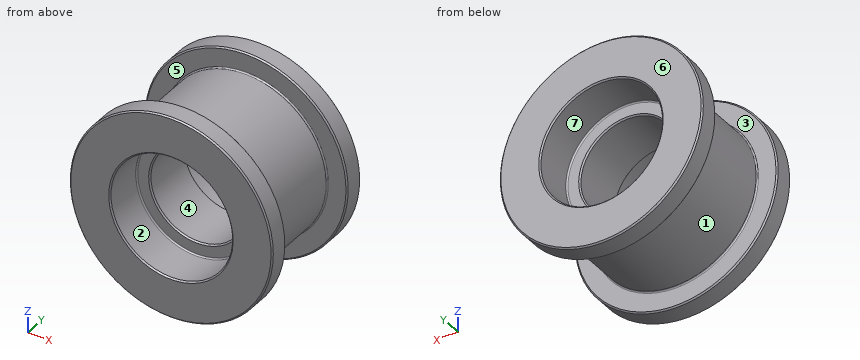
from build123d import *

# Parameters (mm, degrees)
ZKOSEN_1_SIZE = 0.1
ZAOBLIT1_R    = 0.1


with BuildPart() as part:
    # Skica1 → Rotovat1 (revolve)
    with BuildSketch(Plane.XY, mode=Mode.PRIVATE) as rotovat1_sk:
        Polygon((4.5, 10), (7.5, 10), (7.5, 8.5), (6, 8.5), (6, 1.5), (7.5, 1.5), (7.5, 0), (4.5, 0), (4.5, 3), (3.5, 3), (3.5, 7), (4.5, 7), align=None)
    revolve(rotovat1_sk.sketch.rotate(Axis((0, 0, 0), (0, -1, 0)), 90), axis=Axis((0, 0, 0), (0, -1, 0)))

    # Zkosení1
    zkosen_1_edges = [part.edges().sort_by_distance(p)[0] for p in [
        (0, 3, -3.5),
        (0, 0, -4.5),
        (0, 0, -7.5),
        (0, 1.5, -7.5),
        (0, 8.5, -7.5),
        (0, 10, -7.5),
        (0, 10, -4.5),
        (0, 7, -3.5),
    ]]
    chamfer(zkosen_1_edges, length=ZKOSEN_1_SIZE)

    # Zaoblit1
    zaoblit1_edges = [part.edges().sort_by_distance(p)[0] for p in [
        (0, 3, -4.5),
        (0, 1.5, -6),
        (0, 8.5, -6),
        (0, 7, -4.5),
    ]]
    fillet(zaoblit1_edges, radius=ZAOBLIT1_R)


solid = part.part
Source: CAD feature listing. Evaluate the final solid. Frame: model axes, mm. Face numbers are marked on the shaded views. A direction names the side the tool comes from. Round coordinates to 2 decimals unless told otherwise and drop trailing zeros. Write each loop counter-clockwise with the first axis right and the second up, starting at its lowest first coordinate (ties: lowest second). Pieces come first, ordered by that corner, then holes. Notation, with made-up numbers: M 10,22.5 L 19,22.5 A27 ccw 19,45.5 Z; hole C 67.5,69 d4. An arc over 180 degrees is marked long. One line per item, written item: value. Start each with the question number.
Item 1: Mould query, pull axis Z, two halves, no side actions, for the marked faces 1, 2, 3 and 4. Classes: pulls with the +Z half, pulls with the -Z half, needs draft (parallel to the pull), parting line crosses it, or undercut.
Item 2: Pin query (flat end, axial travel): pin 1 (1 mm diameter, centred on x = -4.5, y = 4, fed in from +Z); pin 2 (1.5 mm diameter, centred on x = 3.5, y = 2, fed in from +Z); pin 3 (6 mm diameter, centred on y = 2.5, z = -2, fed in from -X); pin 4 (5.5 mm diameter, centred on x = 0, z = 0, fed in from +Y). Return the tip coordinate at first contact, or that it passes through.
Item 3: Section query B-B (y = 3.5). Return the cut outline in (x, z).
Item 4: Ray query, L1, parallel to X at y = 1.65, z = 0; L2, parallel to X at y = 5.2, z = 0; L3, parallel to Y at x = 6.5, z = 1.25. Return the intervals inside material, ascending. Write a range as from..to.
Item 5: Section query A-A (y = 2). Return the cut outline in (x, z), plus the area to 3 significant figures.
Item 6: Set-up query: the marked faces 5, 6 and 7. Return all of +Z, -Z, +X, -X, +Y, -Y with unobstructed straight access to the full face (end or side cutting, diameter ignored); none if empty.
Result set:
1. face 1: parting line crosses it
1. face 2: undercut
1. face 3: needs draft
1. face 4: undercut
2. pin 1: stops at z = 4.47
2. pin 2: stops at z = 6.85
2. pin 3: stops at x = -7.5
2. pin 4: passes through
3. outline: C 0,0 d12; hole C 0,0 d7
4. L1: x = -6..-4.5, 4.5..6
4. L2: x = -6..-3.5, 3.5..6
4. L3: y = 0..1.5, 8.5..10
5. outline: C 0,0 d12; hole C 0,0 d9
5. area: 49.5 mm²
6. face 5: none
6. face 6: +Z, -Z, +X, -X, +Y
6. face 7: +Y
